from build123d import *

# Parameters (mm, degrees)
BOSS_EXTRUDE1_DEPTH        = 192.05
BOSS_EXTRUDE1_DEPTH_BACK   = 192.05
BOSS_EXTRUDE1_2_DEPTH      = 192.05
BOSS_EXTRUDE1_2_DEPTH_BACK = 192.05
SKETCH3_OUTSIDE_W          = 508.562
SKETCH3_OUTSIDE_H          = 558.651
CUT_EXTRUDE1_DEPTH         = 12
SKETCH4_OUTSIDE_W          = 508.562
SKETCH4_OUTSIDE_H          = 526.289
CUT_EXTRUDE2_DEPTH         = 12
BOSS_EXTRUDE4_START        = 120
BOSS_EXTRUDE4_DEPTH        = 12
BOSS_EXTRUDE10_DEPTH       = 6


with BuildPart() as part:
    # Sketch2 → Boss-Extrude1 (new body, two sides)
    with BuildSketch(Plane(origin=(0, 0, 0), x_dir=(0, 0, -1), z_dir=(1, 0, 0))) as boss_extrude1_sk:
        Polygon((0, 0), (-270.822132078, 47.753248858), (-272.90591021, 35.935555822), (-2.083778132, -11.817693036), align=None)
    extrude(amount=BOSS_EXTRUDE1_DEPTH)
    extrude(boss_extrude1_sk.sketch, amount=-BOSS_EXTRUDE1_DEPTH_BACK)

    # Sketch3 outside → Cut-Extrude1 (cut)
    with BuildSketch(Plane(origin=(0, 0, 0), x_dir=(1, 0, 0), z_dir=(0, 0.984807753, -0.173648178))):
        with Locations((0, -96.4215)):
            Rectangle(SKETCH3_OUTSIDE_W, SKETCH3_OUTSIDE_H)
        with BuildLine():
            Line((0, -275), (112.39737442, -275))
            ThreePointArc((112.39737442, -275), (171.471178999, -248.947063059), (192.068830938, -187.757140317))
            Line((192.068830938, -187.757140317), (181.614285483, -72.757140317))
            ThreePointArc((181.614285483, -72.757140317), (155.889892025, -20.926195422), (101.942828966, 0))
            Line((101.942828966, 0), (-101.942828966, 0))
            ThreePointArc((-101.942828966, 0), (-155.889892025, -20.926195422), (-181.614285483, -72.757140317))
            Line((-181.614285483, -72.757140317), (-192.068830938, -187.757140317))
            ThreePointArc((-192.068830938, -187.757140317), (-171.471178999, -248.947063059), (-112.39737442, -275))
            Line((-112.39737442, -275), (0, -275))
        make_face(mode=Mode.SUBTRACT)
    extrude(amount=-CUT_EXTRUDE1_DEPTH, mode=Mode.SUBTRACT)



with BuildPart() as body_2:
    # Sketch2 → Boss-Extrude1 2 (new body, two sides)
    with BuildSketch(Plane(origin=(0, 0, 0), x_dir=(0, 0, -1), z_dir=(1, 0, 0))) as boss_extrude1_2_sk:
        Polygon((109.404715977, 257.741358967), (62.516980558, 147.280776552), (73.5630388, 142.592003011), (120.450774218, 253.052585425), align=None)
    extrude(amount=BOSS_EXTRUDE1_2_DEPTH)
    extrude(boss_extrude1_2_sk.sketch, amount=-BOSS_EXTRUDE1_2_DEPTH_BACK)

    # Sketch4 outside → Cut-Extrude2 (cut)
    with BuildSketch(Plane(origin=(0, 0, 0), x_dir=(1, 0, 0), z_dir=(0, 0.390731128, 0.920504853))):
        with Locations((0, 83.4025)):
            Rectangle(SKETCH4_OUTSIDE_W, SKETCH4_OUTSIDE_H)
        with BuildLine():
            Line((-112.05, 280), (112.05, 280))
            ThreePointArc((112.05, 280), (168.618542495, 256.568542495), (192.05, 200))
            Line((192.05, 200), (192.05, 190))
            ThreePointArc((192.05, 190), (183.263203436, 168.786796564), (162.05, 160))
            Line((162.05, 160), (-162.05, 160))
            ThreePointArc((-162.05, 160), (-183.263203436, 168.786796564), (-192.05, 190))
            Line((-192.05, 190), (-192.05, 200))
            ThreePointArc((-192.05, 200), (-168.618542495, 256.568542495), (-112.05, 280))
        make_face(mode=Mode.SUBTRACT)
    extrude(amount=-CUT_EXTRUDE2_DEPTH, mode=Mode.SUBTRACT)


with BuildPart() as part_1:
    add(part.part)

    add(body_2.part)  # Boss-Extrude4 merges body 2
    # Sketch6 → Boss-Extrude4 (add)
    with BuildSketch(Plane(origin=(0, 0, 0), x_dir=(0, 0, -1), z_dir=(1, 0, 0)).offset(BOSS_EXTRUDE4_START)):
        with BuildLine():
            Line((-253.20975515, 32.462592269), (-137.494844171, 12.058931393))
            Line((-137.494844171, 12.058931393), (-21.779933192, -8.344729483))
            ThreePointArc((-21.779933192, -8.344729483), (-4.462889813, -36.328759752), (25.301600034, -22.290914988))
            Line((25.301600034, -22.290914988), (91.973135869, 134.777380441))
            ThreePointArc((91.973135869, 134.777380441), (92.106715891, 150.084134879), (81.377661369, 161.00210008))
            Line((81.377661369, 161.00210008), (112.636151649, 234.642488356))
            ThreePointArc((112.636151649, 234.642488356), (132.535530375, 195.215307548), (131.79795497, 151.057139078))
            Line((131.79795497, 151.057139078), (83.48988024, -31.450025326))
            ThreePointArc((83.48988024, -31.450025326), (29.105608653, -96.481302081), (-55.668839629, -96.387117006))
            Line((-55.668839629, -96.387117006), (-203.373392469, -27.062109534))
            ThreePointArc((-203.373392469, -27.062109534), (-234.867841078, -2.805661741), (-253.20975515, 32.462592269))
        make_face()
    boss_extrude4 = extrude(amount=BOSS_EXTRUDE4_DEPTH)

    # Mirror1: Boss-Extrude4 across plane
    add(boss_extrude4.mirror(Plane(origin=(0, 0, 0), x_dir=(0, 0, 1), z_dir=(1, 0, 0))))

    # Sketch27 → Boss-Extrude10 (add, symmetric)
    with BuildSketch(Plane(origin=(68.75, 11.938312215, 67.70553302), x_dir=(0.707106781, -0.122787804, -0.69636424), z_dir=(0.707106781, 0.122787804, 0.69636424))):
        Polygon((52.772817594, -107.537852274), (193.944024949, -293.317225843), (151.463217587, -297.865726007), (-40.700349563, -88.502554793), (-158.448989832, -65.970042163), (-352.630009772, -361.465171741), (-394.307309716, -366.661581013), (-247.22718241, -50.129513852), (-247.22718241, -12.000000012), (52.772817594, -12.000000012), align=None)
    boss_extrude10 = extrude(amount=BOSS_EXTRUDE10_DEPTH, both=True)

    # Mirror3: Boss-Extrude10 across plane
    add(boss_extrude10.mirror(Plane(origin=(0, 0, 0), x_dir=(0, 0, 1), z_dir=(1, 0, 0))))


solid = part_1.part
Model file for the job. Use its own axes, mm. A direction names the side the tool comes from. Round coordinates to 2 decimals unless told otherwise and drop trailing zeros. Order: outer loops, then holes, each group sorted by start corner. A loop starts at its lowest first (then second) coordinate and runs counter-clockwise, first axis right, second up.
(1) Band-saw the part on C-C (y = -246). List the corners of the cut face in (x, z).
(2) Band-saw the part on B-B (y = 56.5). List the corners of the cut face in (x, z), then the cut area to 3 significant figures.
(3) Pull direction X, two halves, no side cores. Call faces 5 (the face through (120, -10, 30)), 6 (the face through (-166.877, 38.208, 250.757)), 7 (the face through (158.74, -155.95, 328.42)), 8 (the face through (-125.92, 55.14, -58.17)): released by +X, released by -X, zero draft, split by the parting line, or undercut.
(4) Drill centre lines: line 1 (Z direction, x = -73, y = 170.5); line 2 (Y direction, x = -37.5, z = 262); line 3 (Z direction, x = 128.5, y = -83.5). Where is each one in solid material? Low to high.
(5) Band-saw the part on D-D (z = -36). List the corners of the cut face in (x, y).
(6) 3-axis set-ups, long thin cutter, end or side, ignore diameter. For faces 1 (the face through (-155.34, -199.18, 17.13)), 2 (the face through (125.92, 55.14, -58.17)), 3 (the face through (125.92, -3.23, 234.51)), 4 (the face through (-97.774, -101.843, 66.913)): which of +Z, -Z, +X, -X, +Y, -Y reach the whole face in a straight line?
(7) Band-saw the part on A-A (x = 68.5). List the corners of the cut face in (y, z).
(8) Pin check, flat tips, straight feed: pin 1 (4 mm diameter, centred on x = -101.5, y = -10.5, fed in from +Z); pin 2 (6 mm diameter, centred on x = -80, z = -65.5, fed in from +Y); pin 3 (4 mm diameter, centred on x = 54, z = 191.5, fed in from -Y). Stop position of each tip, or through.
Verdict:
1. outline: (-194.66, 372.05) - (-156.33, 333.12) - (-148.6, 342.51) - (-186.7, 381.19) - close; (-183.22, 5.57) - (-174, -2.3) - (-139.24, 32.99) - (-148.6, 40.73) - close; (139.24, 32.99) - (174, -2.3) - (183.22, 5.57) - (148.6, 40.73) - close; (148.6, 342.51) - (156.33, 333.12) - (194.66, 372.05) - (186.7, 381.19) - close
2. outline: (-132, -106.77) - (-120, -106.77) - (-120, -58.75) - (-132, -58.75) - close; (120, -106.77) - (132, -106.77) - (132, -58.75) - (120, -58.75) - close
2. area: 1,150 mm2
3. face 5: undercut
3. face 6: released by -X
3. face 7: released by +X
3. face 8: zero draft
4. line 1: z = -85.41 to -72.37
4. line 2: y = 34.01 to 46.2
4. line 3: z = -49.85 to 83.13, 276.21 to 293.44
5. outline: (-132, -92.93) - (-120, -92.93) - (-120, 2.91) - (-132, 2.91) - close; (120, -92.93) - (132, -92.93) - (132, 2.91) - (120, 2.91) - close
6. face 1: -Z, -X
6. face 2: +X, -X
6. face 3: +Z, +X, -Y
6. face 4: none
7. outline: (-126.38, 83.73) - (-1.31, 61.68) - (-11.82, 2.08) - (0, 0) - (47.75, 270.82) - (35.94, 272.91) - (25.43, 213.31) - (-90.14, 233.69) - (-75.11, 213.81) - (22.48, 196.6) - (1.64, 78.39) - (-110.56, 98.17) - close; (142.59, -73.56) - (253.05, -120.45) - (257.74, -109.4) - (147.28, -62.52) - close
8. pin 1: stops at z = 255.21
8. pin 2: stops at y = 161.38
8. pin 3: stops at y = -45.94
